Design review of the part built by this model. Coordinates are the model's own, in mm. A direction names the side the tool comes from. Give positions to 0.01 mm unless a question says otherwise; leave off trailing zeros. Write each loop counter-clockwise with the first axis right and the second up, starting at its lowest first coordinate (ties: lowest second). Pieces come first, ordered by that corner, then holes.
```python
from build123d import *

# Parameters (mm, degrees)
BOSS_EXTRUDE1_DEPTH = 2
SKETCH3_R           = 1.4
BOSS_EXTRUDE3_DEPTH = 5


with BuildPart() as part:
    # Sketch1 → Boss-Extrude1 (new body)
    with BuildSketch(Plane(origin=(0, 0, 0), x_dir=(0, 0, -1), z_dir=(1, 0, 0))):
        with BuildLine():
            Line((-1.5, 0), (-1.5, 60))
            ThreePointArc((-1.5, 60), (0, 61.5), (1.5, 60))
            Line((1.5, 60), (1.5, 0))
            ThreePointArc((1.5, 0), (0, -1.5), (-1.5, 0))
        make_face()
    extrude(amount=BOSS_EXTRUDE1_DEPTH)

    # Sketch3 → Boss-Extrude3 (add)
    with BuildSketch(Plane(origin=(2, 0, 0), x_dir=(0, 0, -1), z_dir=(1, 0, 0))):
        Circle(SKETCH3_R)
    extrude(amount=BOSS_EXTRUDE3_DEPTH)


solid = part.part
```
(1) Consider section A-A, the plane z = 0. Give the boundary of the cut face in (x, y).
Resolved:
outline: (0, -1.5) - (2, -1.5) - (2, -1.4) - (7, -1.4) - (7, 1.4) - (2, 1.4) - (2, 61.5) - (0, 61.5) - close
(2) To check wall thickness, follow L1, parallel to X at y = 27, z = 0.75; L2, parallel to Y at x = 3, z = 0.15; L3, parallel to Y at x = 0.75, z = 0.25. State the ranges of each line that lie inside material, in increasing order.
Resolved:
L1: x = 0 to 2
L2: y = -1.39 to 1.39
L3: y = -1.48 to 61.48
(3) Consider section B-B, the plane x = 2.75. Give the boundary of the cut face in (y, z), then the cut area to 3 significant figures.
Resolved:
outline: circle Ø2.8 at (0, 0)
area: 6.16 mm2
(4) Consider section C-C, the plane y = 56. Give the boundary of the cut face in (x, z).
Resolved:
outline: (0, -1.5) - (2, -1.5) - (2, 1.5) - (0, 1.5) - close
(5) Tool access review of faces 1 (the face through (4.46, 0.06, 1.4)), 2 (the face through (1, 61.5, 0)): name each direction out of +Z, -Z, +X, -X, +Y, -Y from which nothing blocks a thin tool from reaching the whole face with its end or side.
Resolved:
face 1: +X
face 2: +X, -X, +Y
